Read the model definition and answer for the solid it produces. Units are mm, in the model's axes. A direction names the side the tool comes from. Coordinates: 2 decimals unless noted, no trailing zeros. Write each loop counter-clockwise with the first axis right and the second up, starting at its lowest first coordinate (ties: lowest second). Pieces come first, ordered by that corner, then holes.
Item 1: Each of these flat-tipped pins is pushed along its axis until it touches: P1, Ø16, axis at x = -17.53, y = 15.85, coming from the -Z side; P2, Ø1.2, axis at x = -12, z = 1.5, coming from the -Y side; P3, Ø0.9, axis at y = 2.5, z = 3, coming from the -X side; P4, Ø1.5, axis at y = 19.5, z = 2, coming from the -X side. Where does it stop, or does it pass through?
Item 2: Section B-B (y = 11.25) is taken. Give the vertices of the cut face in (x, z).
Item 3: Determine the mould class of faces 1 (the face through (29, 3.379, 2)), 2 (the face through (18.475, 8.895, 1.972)), 3 (the face through (48.512, 15.643, 1.972)) for opening direction Y: released by +Y, released by -Y, zero draft, split by the parting line, or undercut.
Item 4: Section A-A (x = 43.5) is taken. Give the vertices of the cut face in (y, z).
Item 5: Section C-C (z = 2.1) is taken. Give the vertices of the cut face in (x, y).
Item 6: Straight lines are drawn through the part: probe 1 along Y at (x, z) = (19.5, 2.1); probe 2 along Y at (x, z) = (36, 3.4); probe 3 along X at (y, z) = (9, 0.85). For each, find the intervals that lie inside material, in ascending order.
Item 7: Section D-D (x = 32) is taken. Give the vertices of the cut face in (y, z).
Item 8: A tool of negligible diameter and unlimited length cuts with its end or side. For faces 4 (the face through (-0.57, 9.15, 1.97)), 5 (the face through (-3.89, 2, 2)), 6 (the face through (22.11, 2, 2)), from which of +Z, -Z, +X, -X, +Y, -Y can it reach the whole face along a straight path? Write none if from no direction.
from build123d import *

# Parameters (mm, degrees)
SKETCH2_R           = 1
SKETCH2_R_2         = 8
BOSS_EXTRUDE2_DEPTH = 4


with BuildPart() as part:
    # Sketch2 → Boss-Extrude2 (new body)
    with BuildSketch(Plane.XY):
        with BuildLine():
            Line((-18.567970323, 27.379059863), (36.515267991, 27.379059863))
            ThreePointArc((36.515267991, 27.379059863), (48.515267991, 15.379059863), (36.515267991, 3.379059863))
            Line((36.515267991, 3.379059863), (22.110149126, 3.379059863))
            Line((22.110149126, 3.379059863), (22.110149126, 0.351018879))
            Line((22.110149126, 0.351018879), (-3.889850874, 0.351018879))
            Line((-3.889850874, 0.351018879), (-3.889850874, 3.379059863))
            Line((-3.889850874, 3.379059863), (-18.567970323, 3.379059863))
            ThreePointArc((-18.567970323, 3.379059863), (-30.567970323, 15.379059863), (-18.567970323, 27.379059863))
        make_face()
        with Locations((-1.526351166, 22.851018879)):
            Circle(SKETCH2_R, mode=Mode.SUBTRACT)
        with Locations((19.473648834, 22.851018879)):
            Circle(SKETCH2_R, mode=Mode.SUBTRACT)
        with Locations((-1.526351166, 8.851018879)):
            Circle(SKETCH2_R, mode=Mode.SUBTRACT)
        with Locations((19.473648834, 8.851018879)):
            Circle(SKETCH2_R, mode=Mode.SUBTRACT)
        with Locations((8.973648834, 15.851018879)):
            Circle(SKETCH2_R_2, mode=Mode.SUBTRACT)
        with BuildLine():
            ThreePointArc((-10.371103668, 22.836892714), (-25.952222618, 10.465418608), (-8.181666286, 19.411477345))
            ThreePointArc((-8.181666286, 19.411477345), (-3.926588869, 24.543637074), (-10.371103668, 22.836892714))
        make_face(mode=Mode.SUBTRACT)
        with BuildLine():
            ThreePointArc((28.318401336, 8.865145043), (43.899520286, 21.236619149), (26.128963954, 12.290560412))
            ThreePointArc((26.128963954, 12.290560412), (21.873886537, 7.158400683), (28.318401336, 8.865145043))
        make_face(mode=Mode.SUBTRACT)
    extrude(amount=BOSS_EXTRUDE2_DEPTH)


solid = part.part
Established:
1. P1: passes through
1. P2: stops at y = 3.38
1. P3: stops at x = -3.89
1. P4: stops at x = -30.08
2. outline: (-29.84, 0) - (-26.41, 0) - (-26.41, 4) - (-29.84, 4) - close; (-8.65, 0) - (2.43, 0) - (2.43, 4) - (-8.65, 4) - close; (15.52, 0) - (22.11, 0) - (22.11, 4) - (15.52, 4) - close; (44.35, 0) - (47.78, 0) - (47.78, 4) - (44.35, 4) - close
3. face 1: released by -Y
3. face 2: undercut
3. face 3: split by the parting line
4. outline: (5.62, 0) - (9.89, 0) - (9.89, 4) - (5.62, 4) - close; (21.82, 0) - (25.14, 0) - (25.14, 4) - (21.82, 4) - close
5. outline: (-18.57, 3.38) - (-3.89, 3.38) - (-3.89, 0.35) - (22.11, 0.35) - (22.11, 3.38) - (36.52, 3.38) arc R12 ccw to (36.52, 27.38) - (-18.57, 27.38) arc R12 ccw to start; hole (-10.37, 22.84) arc R10 ccw (long way) to (-8.18, 19.41) arc R3.5 ccw (long way) to start; hole circle Ø2 at (-1.53, 8.85); hole circle Ø2 at (-1.53, 22.85); hole circle Ø16 at (8.97, 15.85); hole circle Ø2 at (19.47, 8.85); hole circle Ø2 at (19.47, 22.85); hole (26.13, 12.29) arc R3.5 ccw (long way) to (28.32, 8.87) arc R10 ccw (long way) to start
6. probe 1: y = 0.35 to 7.85, 9.85 to 21.85, 23.85 to 27.38
6. probe 2: y = 3.38 to 5.86, 25.84 to 27.38
6. probe 3: x = -28.73 to -24.81, -10.24 to -2.52, -0.54 to 4.84, 13.1 to 18.48, 20.46 to 21.32, 42.76 to 46.68
7. outline: (3.38, 0) - (6.47, 0) - (6.47, 4) - (3.38, 4) - close; (25.23, 0) - (27.38, 0) - (27.38, 4) - (25.23, 4) - close
8. face 4: +Z, -Z
8. face 5: +Z, -Z, -X, -Y
8. face 6: +Z, -Z, +X, -Y
